Verification items for the finished model (mm, model axes). Face numbers are marked on the shaded views. Give positions to 0.01 mm unless a question says otherwise; leave off trailing zeros. Write each loop counter-clockwise with the first axis right and the second up, starting at its lowest first coordinate (ties: lowest second). Pieces come first, ordered by that corner, then holes. Notation, with made-up numbers: (84, 11) - (117, 11) arc R14 ccw to (117, 31) - close; hole circle Ø7 at (-16, 37). An arc over 180 degrees is marked (long way). Answer as a JSON object with one key per item and string values. Group by question number.
Item 1: Scan lines: line 1 along Y through (x, z) = (0, 1.3); line 2 along Y through (x, z) = (0, -0.9); line 3 along Z through (x, y) = (-16.5, 49.5). Record each from-to range of solid material in increasing order. Write a range as [from, to].
Item 2: Go/stop test with flat-tipped pins: pin 1 (1.6 mm diameter, centred on y = -47, z = 1, fed in from -X); pin 2 (1.6 mm diameter, centred on x = 51, z = 1, fed in from +Y); pin 3 (6 mm diameter, centred on x = 14, y = 42.5, fed in from -Z); pin 4 (1.6 mm diameter, centred on y = 0.5, z = 0.5, fed in from -X). Record where each tip stops, or that it passes through.
Item 3: Sectioned sample at D-D, the plane y = -46.5. Record the boundary of the cut face in (x, z), and give its area (3 significant figures).
Item 4: Sectioned sample at B-B, the plane y = -7. Record the boundary of the cut face in (x, z).
Item 5: Draft check along Y on the marked faces 1 and 2. Enter one of: +Y half, -Y half, draft (parallel to the pull), parting line (faces both ways), or undercut.
Item 6: Sectioned sample at A-A, the plane x = 0. Record the boundary of the cut face in (y, z), and give its area (3 significant figures).
Item 7: Sectioned sample at C-C, the plane z = -2.05. Record the boundary of the cut face in (x, y).
```python
from build123d import *

# Parameters (mm, degrees)
SKETCH1_R           = 63.5
SKETCH1_R_2         = 29.1
SKETCH1_W           = 9.3726
SKETCH1_H           = 6.1976
SKETCH1_W_2         = 6.1976
SKETCH1_H_2         = 9.3726
BOSS_EXTRUDE1_DEPTH = 2
SKETCH2_R           = 61.3
SKETCH2_R_2         = 59.8
BOSS_EXTRUDE2_DEPTH = 3


with BuildPart() as part:
    # Sketch1 → Boss-Extrude1 (new body)
    with BuildSketch(Plane(origin=(0, 0, 0), x_dir=(0, 1, 0), z_dir=(0, 0, 1))):
        with Locations(Location((0, 0, 0), (0, 0, 270))):
            Circle(SKETCH1_R)
        with Locations(Location((0, 0, 0), (0, 0, 270))):
            Circle(SKETCH1_R_2, mode=Mode.SUBTRACT)
        with Locations((48.905920984, 0.073333248)):
            Rectangle(SKETCH1_W, SKETCH1_H, mode=Mode.SUBTRACT)
        with Locations((-0.073333248, 48.905920984)):
            Rectangle(SKETCH1_W_2, SKETCH1_H_2, mode=Mode.SUBTRACT)
        with Locations((0.073333248, -48.905920984)):
            Rectangle(SKETCH1_W_2, SKETCH1_H_2, mode=Mode.SUBTRACT)
        with Locations((-48.905920984, -0.073333248)):
            Rectangle(SKETCH1_W, SKETCH1_H, mode=Mode.SUBTRACT)
    extrude(amount=BOSS_EXTRUDE1_DEPTH)

    # Sketch2 → Boss-Extrude2 (add)
    with BuildSketch(Plane(origin=(0, 0, 0), x_dir=(1, 0, 0), z_dir=(0, 0, -1))):
        Circle(SKETCH2_R)
        with Locations(Location((0, 0, 0), (0, 0, 180))):
            Circle(SKETCH2_R_2, mode=Mode.SUBTRACT)
    extrude(amount=BOSS_EXTRUDE2_DEPTH)


solid = part.part
```
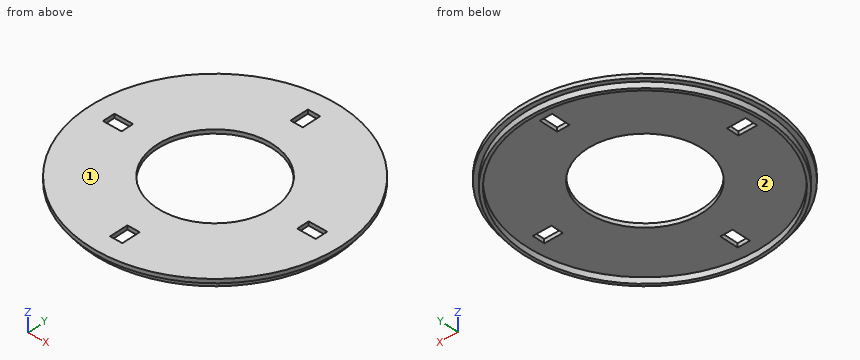
Geometry check:
{
 "1": {"line 1": "[-63.5, -53.59], [-44.22, -29.1], [29.1, 44.22], [53.59, 63.5]", "line 2": "[-61.3, -59.8], [59.8, 61.3]", "line 3": "[0, 2]"},
 "2": {"pin 1": "x = -43.56", "pin 2": "y = 38.89", "pin 3": "z = 0", "pin 4": "x = -63.5"},
 "3": {"outline": "(-43.24, 0) - (-39.94, 0) - (-39.94, -3) - (-37.6, -3) - (-37.6, 0) - (-3.03, 0) - (-3.03, 2) - (-43.24, 2) - close; (3.17, 0) - (37.6, 0) - (37.6, -3) - (39.94, -3) - (39.94, 0) - (43.24, 0) - (43.24, 2) - (3.17, 2) - close", "area": "175 mm^2"},
 "4": {"outline": "(-63.11, 0) - (-60.9, 0) - (-60.9, -3) - (-59.39, -3) - (-59.39, 0) - (-28.25, 0) - (-28.25, 2) - (-63.11, 2) - close; (28.25, 0) - (59.39, 0) - (59.39, -3) - (60.9, -3) - (60.9, 0) - (63.11, 0) - (63.11, 2) - (28.25, 2) - close"},
 "5": {"face 1": "draft", "face 2": "undercut"},
 "6": {"outline": "(-63.5, 0) - (-61.3, 0) - (-61.3, -3) - (-59.8, -3) - (-59.8, 0) - (-53.59, 0) - (-53.59, 2) - (-63.5, 2) - close; (-44.22, 0) - (-29.1, 0) - (-29.1, 2) - (-44.22, 2) - close; (29.1, 0) - (44.22, 0) - (44.22, 2) - (29.1, 2) - close; (53.59, 0) - (59.8, 0) - (59.8, -3) - (61.3, -3) - (61.3, 0) - (63.5, 0) - (63.5, 2) - (53.59, 2) - close", "area": "109 mm^2"},
 "7": {"outline": "circle Ø122.6 at (0, 0); hole circle Ø119.6 at (0, 0)"}
}
